```python
from build123d import *

# Parameters (mm, degrees)
F0_W         = 400
F0_H         = 100
F1_DEPTH     = 50
F2_R         = 5
F3_T1_DEPTH  = 57.5
F3_T3_DEPTH  = 90
F3_S7_W      = 5
F3_S7_H      = 5
F3_T8_DEPTH  = 5
F3_T12_ANGLE = 90
F4_R         = 10
F5_DEPTH     = 50.001


# Not quite as in the source:
# - a fillet or chamfer that OpenCascade refuses, or shapes differently, is made with other operations: its cross-section is extruded or revolved along the edge and cut away or added


with BuildPart() as f1:
    # F0 (on Top) → F1 (new body)
    with BuildSketch(Plane.XY):
        with Locations((-0.9229257703, 15.3983329495)):
            Rectangle(F0_W, F0_H)
    extrude(amount=F1_DEPTH)

    # F2
    f2_edges = [f1.edges().sort_by_distance(p)[0] for p in [
        (-200.922926, -34.601667, 25),
        (199.077074, -34.601667, 25),
        (199.077074, 65.398333, 25),
        (199.077074, 15.398333, 50),
        (-0.922926, -34.601667, 50),
        (-0.922926, 65.398333, 50),
    ]]
    fillet(f2_edges, radius=F2_R)

    # F3: fillet of radius 5 on 1 edges, made by hand

    # F3_s2 → F3_t1 (cut)
    with BuildSketch(Plane.XY.offset(-12.5)):
        with BuildLine():
            ThreePointArc((-195.9229257703, 65.3983329495), (-199.4584596762, 63.9338668555), (-200.9229257703, 60.3983329495))
            Line((-200.9229257703, 60.3983329495), (-200.9229257703, 65.3983329495))
            Line((-200.9229257703, 65.3983329495), (-195.9229257703, 65.3983329495))
        make_face()
    extrude(amount=F3_T1_DEPTH, mode=Mode.SUBTRACT)

    # F3_s4 → F3_t3 (cut)
    with BuildSketch(Plane.XZ.offset(-60.3983329495)):
        with BuildLine():
            ThreePointArc((-200.9229257703, 45), (-199.4584596762, 48.5355339059), (-195.9229257703, 50))
            Line((-195.9229257703, 50), (-200.9229257703, 50))
            Line((-200.9229257703, 50), (-200.9229257703, 45))
        make_face()
    extrude(amount=F3_T3_DEPTH, mode=Mode.SUBTRACT)


with BuildPart() as f3_tool6:
    # F3_s7 → F3_t8 (new body)
    with BuildSketch(Plane.YZ.offset(-195.9229257703)):
        with Locations((-32.1016670505, 47.5)):
            Rectangle(F3_S7_W, F3_S7_H)
    extrude(amount=-F3_T8_DEPTH)

    # F3_s9 → F3_t10 (revolve, cut)
    with BuildSketch(Plane(origin=(-195.9229257703, -29.6016670505, 45), x_dir=(0, 0.7071067812, -0.7071067812), z_dir=(0, 0.7071067812, 0.7071067812))):
        with BuildLine():
            ThreePointArc((0, -5), (5, 0), (0, 5))
            Line((0, 5), (0, -5))
        make_face()
    revolve(axis=Axis((-195.9229257703, -29.6016670505, 45), (-1, 0, 0)), mode=Mode.SUBTRACT)


with BuildPart() as f1_1:
    add(f1.part)

    # F3_t5: cut F3_tool6
    add(f3_tool6.part, mode=Mode.SUBTRACT)

    # F3_s11 → F3_t12 (revolve, cut)
    with BuildSketch(Plane.XY.offset(45)):
        with BuildLine():
            ThreePointArc((-200.9229257703, 60.3983329495), (-199.4584596762, 63.9338668555), (-195.9229257703, 65.3983329495))
            Line((-195.9229257703, 65.3983329495), (-200.9229257703, 65.3983329495))
            Line((-200.9229257703, 65.3983329495), (-200.9229257703, 60.3983329495))
        make_face()
    revolve(axis=Axis((-200.9229257703, 60.3983329495, 45), (1, 0, 0)), revolution_arc=F3_T12_ANGLE, mode=Mode.SUBTRACT)

    # F4 (on face) → F5 (cut, through all)
    with BuildSketch(Plane.XY.offset(50)):
        with Locations((149.0770742297, 15.3983329495)):
            Circle(F4_R)
    extrude(amount=-F5_DEPTH, mode=Mode.SUBTRACT)


solid = f1_1.part
```
Geometry check sheet. Reference: the model listing, model coordinates, mm. Round coordinates to 2 decimals unless told otherwise and drop trailing zeros. Order: outer loops, then holes, each group sorted by start corner. A loop starts at its lowest first (then second) coordinate and runs counter-clockwise, first axis right, second up. Notation, with made-up numbers: (5, 3) -> (42, 3) arc R24 cw to (42, 33) -> close; hole circle Ø2 at (-6.75, 13.25). An arc over 180 degrees is marked (long way). Return JSON: item names as keys, results as strings. Group by question number.
Q1. Material ranges on probe 1 along X at (y, z) = (14.5, 5); probe 2 along X at (y, z) = (17.5, 14); probe 3 along Y at (x, z) = (155.5, 43), recorded low to high. Write a range as from..to.
Q2. Release check for a two-part mould opening along X. For faces 1 (the flat face through (-200.923, 15, 22)), 2 (the cylindrical face through (158.315, 11.568, 25.35)), 3 (the flat face through (199.077, 15, 22)), 4 (the flat face through (-4, 16, 50)) record: released by +X, released by -X, zero draft, split by the parting line, or undercut.
Q3. Section check A-A, the plane y = 20. Record the boundary of the cut face in (x, z), plus the area to 3 significant figures.
Q4. Gauge pin test, flat end, axial feed: pin 1 (12 mm diameter, centred on x = 149.08, y = 15.4, fed in from +Z). Record the tip position at first contact, or that the pin passes through.
Numbers:
{
 "1": {"probe 1": "-200.92..139.12, 159.04..199.08", "probe 2": "-200.92..139.3, 158.85..199.08", "probe 3": "-34.6..7.73, 23.06..65.4"},
 "2": {"face 1": "released by -X", "face 2": "undercut", "face 3": "released by +X", "face 4": "zero draft"},
 "3": {"outline": "(-200.92, 0) -> (140.2, 0) -> (140.2, 50) -> (-195.92, 50) arc R5 ccw to (-200.92, 45) -> close; (157.96, 0) -> (199.08, 0) -> (199.08, 45) arc R5 ccw to (194.08, 50) -> (157.96, 50) -> close", "area": "19,100 mm^2"},
 "4": {"pin 1": "through"}
}
